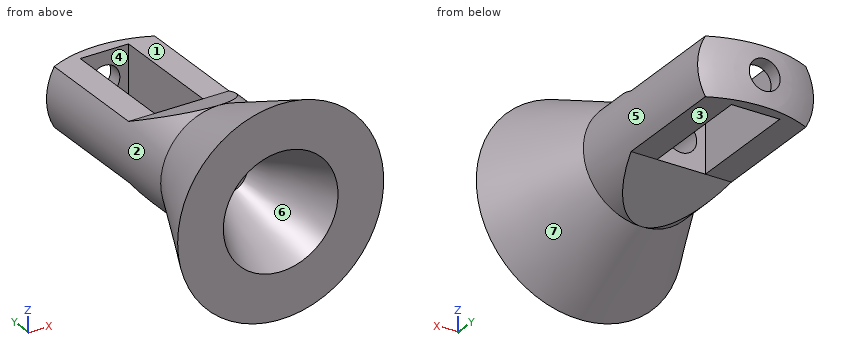
```python
from build123d import *

# Parameters (mm, degrees)
F3_DEPTH = 30
F5_W     = 25
F5_H     = 60
F6_DEPTH = 68.316383


with BuildPart() as f1:
    # F0 (on Top) → F1 (revolve)
    with BuildSketch(Plane.XY):
        with BuildLine():
            Line((-30, 50), (-53.315383, 0))
            Line((-53.315383, 0), (-29.677889, 0))
            Line((-29.677889, 0), (-10, 42.19937))
            Line((-10, 42.19937), (-8, 42.19937))
            Line((-8, 42.19937), (-8, 149.473135))
            ThreePointArc((-8, 149.473135), (-19.353102, 146.848573), (-30, 142.113087))
            Line((-30, 142.113087), (-30, 50))
        make_face()
    revolve(axis=Axis((0, 44.812715, 0), (0, 1, 0)))

    # F2 (on Right) → F3 (cut, symmetric)
    with BuildSketch(Plane.YZ):
        Polygon((149.473135, 30), (50, 30), (82.167604, 15), (149.473135, 15), align=None)
    extrude(amount=F3_DEPTH, both=True, mode=Mode.SUBTRACT)

    # F4: F1 across plane


with BuildPart() as f1_1:
    add(f1.part)
    add(f1.part.mirror(Plane.XY), mode=Mode.INTERSECT)

    # F5 (on face) → F6 (cut, through all)
    with BuildSketch(Plane.XY.offset(15)):
        with Locations((0, 112.167604)):
            Rectangle(F5_W, F5_H)
    extrude(amount=-F6_DEPTH, mode=Mode.SUBTRACT)


solid = f1_1.part
```
Geometry check sheet. Reference: the model listing, model coordinates, mm. Face numbers are marked on the shaded views. A direction names the side the tool comes from. Round coordinates to 2 decimals unless told otherwise and drop trailing zeros. Loops run counter-clockwise (first coordinate to the right, second up) from the corner with the lowest first, then second, coordinate; pieces in that order, holes last. Notation, with made-up numbers: M 64.25,-10 L 72.25,-10 A33 ccw 72.25,19 Z; hole C 76,9.25 d1. An arc over 180 degrees is marked long. Return JSON: item names as keys, results as strings. Group by question number.
(1) Section check A-A, the plane y = 91.5. Enter the section's corners in (x, z), and give its area (3 significant figures).
(2) Section check C-C, the plane y = 47. Enter the section's corners in (x, z), and give its area (3 significant figures).
(3) Mould release check, pull along X, two halves, no side actions. Record for the marked faces 5, 6 and 7: pulls with the +X half, pulls with the -X half, needs draft (parallel to the pull), parting line crosses it, or undercut.
(4) Section check B-B, the plane y = 16.5. Enter the section's corners in (x, z).
(5) Go/stop test with flat-tipped pins: pin 1 (4 mm diameter, centred on y = 30, z = -18, fed in from -X); pin 2 (16 mm diameter, centred on x = 0, z = 0.5, fed in from -Y); pin 3 (10 mm diameter, centred on x = -12, z = -41.5, fed in from +Y). Record where each tip stops, or that it passes through.
(6) Set-up check for the marked faces 1, 2, 3 and 4: record each of +Z, -Z, +X, -X, +Y, -Y from which the full face is reachable in a straight line by a thin tool's end or side.
(7) Scan lines: line 1 along Z through (x, y) = (0, 147.5); line 2 along X through (y, z) = (114, -5); line 3 along Z through (x, y) = (0, 63.5). Record each from-to range of solid material in increasing order. Write a range as [from, to].
Data:
{
 "1": {"outline": "M -25.98,-15 L -12.5,-15 L -12.5,15 L -25.98,15 A30 ccw Z; M 12.5,-15 L 25.98,-15 A30 ccw 25.98,15 L 12.5,15 Z", "area": "972 mm²"},
 "2": {"outline": "C 0,0 d62.8; hole C 0,0 d16", "area": "2,900 mm²"},
 "3": {"face 5": "pulls with the +X half", "face 6": "undercut", "face 7": "parting line crosses it"},
 "4": {"outline": "C 0,0 d91.24; hole C 0,0 d43.97"},
 "5": {"pin 1": "x = -36.39", "pin 2": "y = 42.2", "pin 3": "y = 32.41"},
 "6": {"face 1": "+Z, +X, -X, +Y", "face 2": "-X, +Y", "face 3": "-Z, +X, -X, +Y", "face 4": "+Z, -Z"},
 "7": {"line 1": "[-15, -8], [8, 15]", "line 2": "[-29.58, -12.5], [12.5, 29.58]", "line 3": "[-23.7, -8], [8, 23.7]"}
}
